Input: dimensioned drawing with shaded views. Units: mm. Origin: part minimum x, y, z. A direction names the side the tool comes from. Round coordinates to 2 decimals unless told otherwise and drop trailing zeros. Loops run counter-clockwise (first coordinate to the right, second up) from the corner with the lowest first, then second, coordinate; pieces in that order, holes last. Notation, with made-up numbers: M -23.5,86 L -9.5,86 A33 cw -9.5,120 Z; hole C 1.5,5 d11. An arc over 180 degrees is marked long. Answer as a JSON object with one key per item and string values.
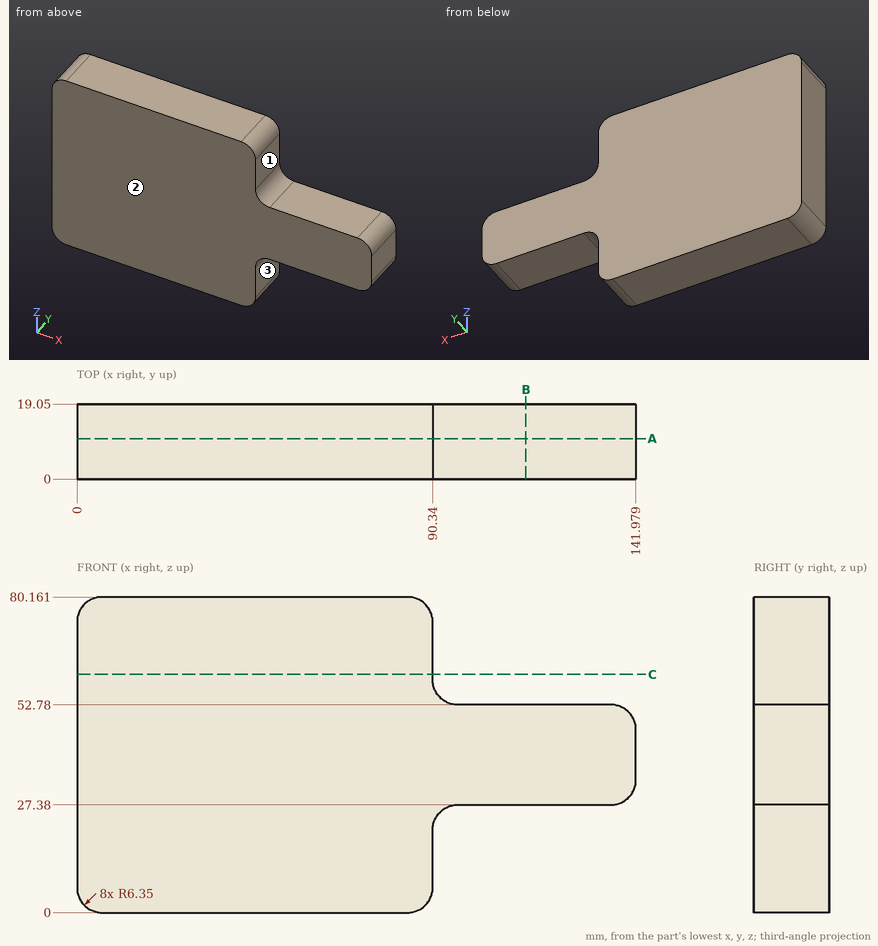
Item 1: Section B-B on x = 114. Return the cut outline in (y, z), then the cut area to 3 significant figures.
Answer sheet:
{"outline": "M 0,27.38 L 19.05,27.38 L 19.05,52.78 L 0,52.78 Z", "area": "484 mm²"}
Item 2: Section C-C on z = 60.5. Return the cut outline in (x, y).
Answer sheet:
{"outline": "M 0,0 L 90.34,0 L 90.34,19.05 L 0,19.05 Z"}
Item 3: Contact query for flat-ended pins moving along their axis: pin 1 Ø6 at (x, y) = (46, 3.5) entering from -Z; pin 2 Ø7.5 at (y, z) = (10.5, 13) entering from +X; pin 3 Ø5.5 at (x, y) = (121, 6) entering from +Z; pin 4 Ø9.5 at (x, y) = (123.5, 11.5) entering from -Z. Output: stop coordinate, or through.
Answer sheet:
{"pin 1": "stops at z = 0", "pin 2": "stops at x = 90.34", "pin 3": "stops at z = 52.78", "pin 4": "stops at z = 27.38"}
Item 4: Line query: probe 1 along X at (y, z) = (4, 19.5); probe 2 along Z at (x, y) = (100, 17.75); probe 3 along Z at (x, y) = (88.5, 2.5). Output: solid intervals per line, ascending. Write a range as from..to.
Answer sheet:
{"probe 1": "x = 0..90.34", "probe 2": "z = 27.38..52.78", "probe 3": "z = 1.88..78.28"}
Item 5: Access query for the marked faces 1, 2 and 3. Directions: +Z, -Z, +X, -X, +Y, -Y. A direction counts if a zero-diameter tool reaches every point of the face in a straight line with its end or side. Return the directions, or none.
Answer sheet:
{"face 1": "+Z, +X, +Y, -Y", "face 2": "+Z, -Z, +X, -X, -Y", "face 3": "-Z, +X, +Y, -Y"}
Item 6: Section A-A on y = 10.25. Return the cut outline in (x, z), then the cut area to 3 significant figures.
Answer sheet:
{"outline": "M 0,6.35 A6.35 ccw 6.35,0 L 83.99,0 A6.35 ccw 90.34,6.35 L 90.34,21.03 A6.35 cw 96.69,27.38 L 135.63,27.38 A6.35 ccw 141.98,33.73 L 141.98,46.43 A6.35 ccw 135.63,52.78 L 96.69,52.78 A6.35 cw 90.34,59.13 L 90.34,73.81 A6.35 ccw 83.99,80.16 L 6.35,80.16 A6.35 ccw 0,73.81 Z", "area": "8,520 mm²"}
